```python
from build123d import *

# Parameters (mm, degrees)
F0_R      = 10.5
F1_DEPTH  = 42
F2_R      = 5
F2_R_2    = 3.5
F3_DEPTH  = 10
F4_W      = 40.5
F4_H      = 42
F4_R      = 7.5
F5_DEPTH  = 20
F6_R      = 3.5
F7_DEPTH  = 21
F8_R      = 16
F9_DEPTH  = 150
F10_SIZE  = 2
F11_R     = 2
F12_DEPTH = 25
F13_R     = 2
F14_DEPTH = 25
F15_R     = 16
F15_R_2   = 7.5
F16_DEPTH = 20


with BuildPart() as f1:
    # F0 (on Right) → F1 (new body)
    with BuildSketch(Plane.YZ):
        Polygon((-20.6668798583, -21.3465905736), (-48.7248089568, 7.8459214502), (-112.5, -74.2), (-112.5, -116.2), align=None)
        Polygon((-35.5, -116.2), (11.8957703927, -55.2259818731), (-20.6668798583, -21.3465905736), (-112.5, -116.2), align=None)
        with BuildLine():
            Line((-12.2649513369, 12.6683319586), (-30.4089327146, 31.4090487239))
            Line((-30.4089327146, 31.4090487239), (-48.7248089568, 7.8459214502))
            Line((-48.7248089568, 7.8459214502), (-20.6668798583, -21.3465905736))
            Line((-20.6668798583, -21.3465905736), (-12.2649513369, -12.6683319586))
            ThreePointArc((-12.2649513369, -12.6683319586), (-12.5145841676, -7.5654843472), (-7.4063318963, -7.6499179231))
            Line((-7.4063318963, -7.6499179231), (0, 0))
            Line((0, 0), (-7.4063318963, 7.6499179231))
            ThreePointArc((-7.4063318963, 7.6499179231), (-12.5145841676, 7.5654843472), (-12.2649513369, 12.6683319586))
        make_face()
        with BuildLine():
            Line((11.8957703927, -55.2259818731), (30.4089327146, -31.4090487239))
            Line((30.4089327146, -31.4090487239), (12.2649513369, -12.6683319586))
            ThreePointArc((12.2649513369, -12.6683319586), (7.4854158324, -12.4345156528), (7.4063318963, -7.6499179231))
            Line((7.4063318963, -7.6499179231), (0, 0))
            Line((0, 0), (-7.4063318963, -7.6499179231))
            ThreePointArc((-7.4063318963, -7.6499179231), (-6.7344343244, -8.7406029941), (-6.5, -10))
            ThreePointArc((-6.5, -10), (-8.5298519937, -13.1762658641), (-12.2649513369, -12.6683319586))
            Line((-12.2649513369, -12.6683319586), (-20.6668798583, -21.3465905736))
            Line((-20.6668798583, -21.3465905736), (11.8957703927, -55.2259818731))
        make_face()
        with BuildLine():
            Line((20.6668798583, 21.3465905736), (-11.8957703927, 55.2259818731))
            Line((-11.8957703927, 55.2259818731), (-30.4089327146, 31.4090487239))
            Line((-30.4089327146, 31.4090487239), (-12.2649513369, 12.6683319586))
            ThreePointArc((-12.2649513369, 12.6683319586), (-8.5298519937, 13.1762658641), (-6.5, 10))
            ThreePointArc((-6.5, 10), (-6.7344343244, 8.7406029941), (-7.4063318963, 7.6499179231))
            Line((-7.4063318963, 7.6499179231), (0, 0))
            Line((0, 0), (7.4063318963, 7.6499179231))
            ThreePointArc((7.4063318963, 7.6499179231), (7.4854158324, 12.4345156528), (12.2649513369, 12.6683319586))
            Line((12.2649513369, 12.6683319586), (20.6668798583, 21.3465905736))
        make_face()
        with BuildLine():
            Line((30.4089327146, -31.4090487239), (48.7248089568, -7.8459214502))
            Line((48.7248089568, -7.8459214502), (20.6668798583, 21.3465905736))
            Line((20.6668798583, 21.3465905736), (12.2649513369, 12.6683319586))
            ThreePointArc((12.2649513369, 12.6683319586), (13.1762658641, 11.4701480063), (13.5, 10))
            ThreePointArc((13.5, 10), (11.2593970059, 6.7344343244), (7.4063318963, 7.6499179231))
            Line((7.4063318963, 7.6499179231), (0, 0))
            Line((0, 0), (7.4063318963, -7.6499179231))
            ThreePointArc((7.4063318963, -7.6499179231), (11.2593970059, -6.7344343244), (13.5, -10))
            ThreePointArc((13.5, -10), (13.1762658641, -11.4701480063), (12.2649513369, -12.6683319586))
            Line((12.2649513369, -12.6683319586), (30.4089327146, -31.4090487239))
        make_face()
        with BuildLine():
            Line((112.5, 74.2), (112.5, 116.2))
            Line((112.5, 116.2), (97.0512585066, 100.2431665641))
            ThreePointArc((97.0512585066, 100.2431665641), (98.4958715968, 97.9032906985), (99, 95.2))
            ThreePointArc((99, 95.2), (94.6458584105, 88.391654029), (86.6390467037, 89.4885086842))
            Line((86.6390467037, 89.4885086842), (20.6668798583, 21.3465905736))
            Line((20.6668798583, 21.3465905736), (48.7248089568, -7.8459214502))
            Line((48.7248089568, -7.8459214502), (112.5, 74.2))
        make_face()
        with BuildLine():
            Line((97.0512585066, 100.2431665641), (112.5, 116.2))
            Line((112.5, 116.2), (35.5, 116.2))
            Line((35.5, 116.2), (-11.8957703927, 55.2259818731))
            Line((-11.8957703927, 55.2259818731), (20.6668798583, 21.3465905736))
            Line((20.6668798583, 21.3465905736), (86.6390467037, 89.4885086842))
            ThreePointArc((86.6390467037, 89.4885086842), (86.1116053551, 100.4168192561), (97.0512585066, 100.2431665641))
        make_face()
        with Locations((56.5, 95.2)):
            Circle(F0_R, mode=Mode.SUBTRACT)
    extrude(amount=F1_DEPTH)

    # F2 (on face) → F3 (cut)
    with BuildSketch(Plane.YZ.offset(42)):
        with Locations((10, -10)):
            Circle(F2_R)
        with Locations((10, -10)):
            Circle(F2_R_2, mode=Mode.SUBTRACT)
        with Locations((-10, -10)):
            Circle(F2_R)
        with Locations((-10, -10)):
            Circle(F2_R_2, mode=Mode.SUBTRACT)
        with Locations((-10, 10)):
            Circle(F2_R)
        with Locations((-10, 10)):
            Circle(F2_R_2, mode=Mode.SUBTRACT)
        with Locations((10, 10)):
            Circle(F2_R)
        with Locations((10, 10)):
            Circle(F2_R_2, mode=Mode.SUBTRACT)
    extrude(amount=-F3_DEPTH, mode=Mode.SUBTRACT)

    # F4 (on face) → F5 (cut)
    with BuildSketch(Plane.YZ.offset(42)):
        with Locations((92.25, 95.2)):
            Rectangle(F4_W, F4_H)
        with Locations((91.5, 95.2)):
            Circle(F4_R, mode=Mode.SUBTRACT)
    extrude(amount=-F5_DEPTH, mode=Mode.SUBTRACT)

    # F6 (on face) → F7 (cut)
    with BuildSketch(Plane(origin=(0, 0, 0), x_dir=(0, -1, 0), z_dir=(-1, 0, 0))):
        Polygon((11.1386554622, 56.2), (-98.5084033613, 56.2), (-11.1386554622, -56.2), (98.5084033613, -56.2), align=None)
        with Locations((-10, -10)):
            Circle(F6_R, mode=Mode.SUBTRACT)
        with Locations((10, -10)):
            Circle(F6_R, mode=Mode.SUBTRACT)
        with Locations((-10, 10)):
            Circle(F6_R, mode=Mode.SUBTRACT)
        with Locations((10, 10)):
            Circle(F6_R, mode=Mode.SUBTRACT)
    extrude(amount=-F7_DEPTH, mode=Mode.SUBTRACT)

    # F8 (on face) → F9 (cut)
    with BuildSketch(Plane.XZ.offset(112.5)):
        with Locations((21, -95.2)):
            Circle(F8_R)
    extrude(amount=-F9_DEPTH, mode=Mode.SUBTRACT)

    # F10
    f10_edges = [f1.edges().sort_by_distance(p)[0] for p in [
        (42, -74, -116.2),
        (42, 92.25, 74.2),
        (42, 72, 95.2),
        (42, 53.75, 116.2),
        (0, -74, -116.2),
        (0, -43.684874, -56.2),
        (0, 43.684874, 56.2),
        (0, 74, 116.2),
    ]]
    chamfer(f10_edges, length=F10_SIZE)

    # F11 (on face) → F12 (cut)
    with BuildSketch(Plane(origin=(0, 0, -116.2), x_dir=(1, 0, 0), z_dir=(0, 0, -1))):
        with Locations((21, 50.5)):
            Circle(F11_R)
        with Locations((21, 91.5)):
            Circle(F11_R)
    extrude(amount=-F12_DEPTH, mode=Mode.SUBTRACT)

    # F13 (on face) → F14 (cut)
    with BuildSketch(Plane.XY.offset(116.2)):
        with Locations((5, 56.5)):
            Circle(F13_R)
        with Locations((15, 91.5)):
            Circle(F13_R)
        with Locations((5, 91.5)):
            Circle(F13_R)
    extrude(amount=-F14_DEPTH, mode=Mode.SUBTRACT)

    # F15 (on face) → F16 (cut)
    with BuildSketch(Plane(origin=(0, 0, 0), x_dir=(0, -1, 0), z_dir=(-1, 0, 0))):
        with Locations((-91.5, 95.2)):
            Circle(F15_R)
        with Locations((-91.5, 95.2)):
            Circle(F15_R_2, mode=Mode.SUBTRACT)
    extrude(amount=-F16_DEPTH, mode=Mode.SUBTRACT)


solid = f1.part
```
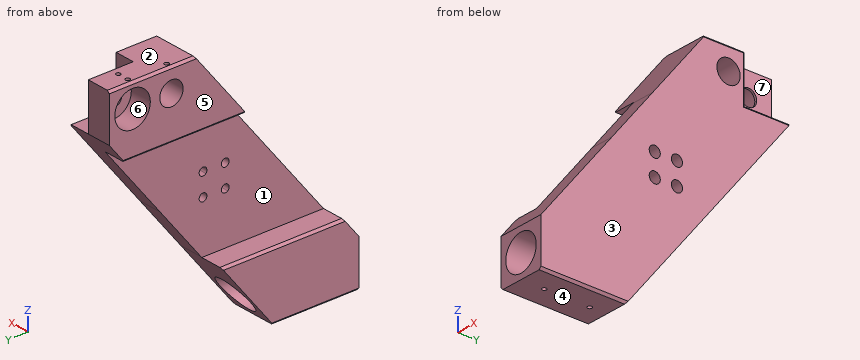
CAD build for the part. Positions are in the model's coordinates, mm. Face numbers are marked on the shaded views. A direction names the side the tool comes from. Round coordinates to 2 decimals unless told otherwise and drop trailing zeros. Order: outer loops, then holes, each group sorted by start corner. A loop starts at its lowest first (then second) coordinate and runs counter-clockwise, first axis right, second up.
Q1. Two-plate mould, pull along Z, no slides. Class the marked faces 1, 2, 3 and 4: pulls with the +Z half, pulls with the -Z half, needs draft (parallel to the pull), parting line crosses it, or undercut.
Q2. Slice it at A-A (x = 26.5). Write the cut outline in (y, z), and give its area (3 significant figures).
Q3. Slice it at B-B (y = -56.5). Write the cut outline in (x, z), and give its area (3 significant figures).
Q4. Drop flat-ended pins along their axis: pin 1 (5 mm diameter, centred on x = 18, y = -77, fed in from +Z); pin 2 (6 mm diameter, centred on x = 28.5, y = 18, fed in from +Z); pin 3 (2.5 mm diameter, centred on x = 5, y = 91.5, fed in from -Z). Give the stop position or say it passes through.
Q5. Wall check: L1, parallel to X at y = -80, z = -95; L2, parallel to X at y = 56.5, z = 112.25; L3, parallel to Y at x = 4.5, z = 99. Give the ranges that are in metal, low to high.
Q6. Slice it at D-D (y = -2). Write the cut outline in (x, z), and give its area (3 significant figures).
Q7. Slice it at C-C (z = -95.2). Write the cut outline in (x, y), and give its area (3 significant figures).
Q8. Which spindle directions (+Z, -Z, +X, -X, +Y, -Y) get a long thin tool onto all of the face, cutting with end or side? Do the marked faces 5, 6 and 7. Say none if no direction does.
Results below:
1. face 1: undercut
1. face 2: pulls with the +Z half
1. face 3: needs draft
1. face 4: pulls with the -Z half
2. outline: (-112.5, -116.2) - (-35.5, -116.2) - (-30.86, -110.22) - (-112.5, -110.22) - close; (-112.5, -80.18) - (-7.5, -80.18) - (112.5, 74.2) - (72, 74.2) - (72, 116.2) - (35.5, 116.2) - (-112.5, -74.2) - close; hole circle Ø7 at (-10, -10); hole circle Ø7 at (-10, 10); hole circle Ø7 at (10, -10); hole circle Ø7 at (10, 10); hole circle Ø21 at (56.5, 95.2)
2. area: 19,100 mm2
3. outline: (0, -114.2) - (2, -116.2) - (40, -116.2) - (42, -114.2) - (42, -2.16) - (21, -2.16) - (21, -56.2) - (2, -56.2) - (0, -58.2) - close; hole circle Ø32 at (21, -95.2)
3. area: 2,840 mm2
4. pin 1: stops at z = -56.2
4. pin 2: stops at z = 97.55
4. pin 3: stops at z = 56.2
5. L1: x = 0 to 5, 37 to 42
5. L2: x = 0 to 3, 7 to 42
5. L3: y = 22.13 to 46.71, 66.29 to 75.96, 107.04 to 112.5
6. outline: (0, -73.1) - (42, -73.1) - (42, 67.96) - (0, 67.96) - (0, 58.2) - (2, 56.2) - (21, 56.2) - (21, -56.2) - (2, -56.2) - (0, -58.2) - close
6. area: 3,560 mm2
7. outline: (0, -112.5) - (5, -112.5) - (5, -19.18) - (0, -19.18) - close; (37, -112.5) - (42, -112.5) - (42, -19.18) - (37, -19.18) - close
7. area: 933 mm2
8. face 5: +Z, -Z, -X, +Y, -Y
8. face 6: -X
8. face 7: +Z, +X, +Y
